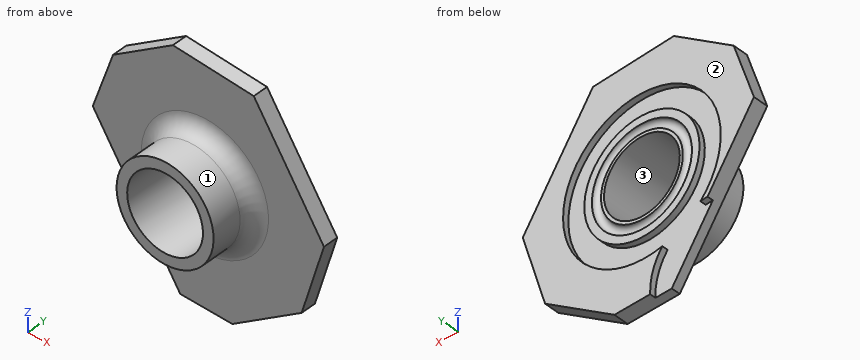
from build123d import *

# Parameters (mm, degrees)
SKETCH_1_R            = 40
SKETCH_1_R_2          = 12.5
EXTRUDE_1_DEPTH       = 20
SKETCH_6_R            = 1.5
SKETCH_12_R           = 43.016285751
SKETCH_12_R_2         = 16
CUT_EXTRUDE_5_DEPTH   = 15
FILLET_2_R            = 5
SKETCH_14_R           = 25.999999999
SKETCH_14_R_2         = 18.999999999
CUT_EXTRUDE_3_DEPTH   = 2
CUT_EXTRUDE_4_DEPTH   = 2
CUT_EXTRUDE_5_2_DEPTH = 10


with BuildPart() as part:
    # Эскиз1 → Вытянуть1 (new body)
    with BuildSketch(Plane(origin=(0, 0, 0), x_dir=(1, 0, 0), z_dir=(0, 1, 0))):
        with Locations(Location((0, 0, 0), (0, 0, 270))):
            Circle(SKETCH_1_R)
        with Locations(Location((0, 0, 0), (0, 0, 270))):
            Circle(SKETCH_1_R_2, mode=Mode.SUBTRACT)
    extrude(amount=EXTRUDE_1_DEPTH)

    # Вырез-По траектории3: sweep along a path in Эскиз4
    with BuildLine(Plane(origin=(0, 20, 0), x_dir=(1, 0, 0), z_dir=(0, 1, 0))) as sweep_3_path:
        CenterArc((0, 0), 15, 0, 360)
    # Эскиз6 → Вырез-По траектории3 (sweep, cut)
    with BuildSketch(Plane(origin=(0, 0, 0), x_dir=(0, 0, -1), z_dir=(1, 0, 0))):
        with Locations((-15, 20)):
            Circle(SKETCH_6_R)
    sweep(path=sweep_3_path.line, mode=Mode.SUBTRACT)

    # Эскиз12 → Cut-Extrude 5 (cut)
    with BuildSketch(Plane.XZ):
        Circle(SKETCH_12_R)
        with Locations(Location((0, 0, 0), (0, 0, 270))):
            Circle(SKETCH_12_R_2, mode=Mode.SUBTRACT)
    extrude(amount=-CUT_EXTRUDE_5_DEPTH, mode=Mode.SUBTRACT)

    # Скругление2
    fillet_2_edges = [part.edges().sort_by_distance(p)[0] for p in [
        (0, 15, 16),
    ]]
    fillet(fillet_2_edges, radius=FILLET_2_R)

    # Эскиз14 → Вырез-Вытянуть3 (cut)
    with BuildSketch(Plane(origin=(0, 20, 0), x_dir=(1, 0, 0), z_dir=(0, 1, 0))):
        with Locations(Location((1.01e-07, 8.4e-08, 0), (0, 0, 270))):
            Circle(SKETCH_14_R)
        with Locations(Location((1.01e-07, 8.4e-08, 0), (0, 0, 270))):
            Circle(SKETCH_14_R_2, mode=Mode.SUBTRACT)
    extrude(amount=-CUT_EXTRUDE_3_DEPTH, mode=Mode.SUBTRACT)

    # Эскиз15 → Вырез-Вытянуть4 (cut)
    with BuildSketch(Plane(origin=(0, 20, 0), x_dir=(1, 0, 0), z_dir=(0, 1, 0))):
        with BuildLine():
            ThreePointArc((-27.297327545, 17.627292527), (-13.760291037, 55.089119116), (-35.71683723, 21.854349851))
            ThreePointArc((-35.71683723, 21.854349851), (-36.252930678, 10.287976674), (-27.297327545, 17.627292527))
        make_face()
    extrude(amount=-CUT_EXTRUDE_4_DEPTH, mode=Mode.SUBTRACT)

    # Эскиз16 → Cut-Extrude 5 2 (cut)
    with BuildSketch(Plane(origin=(0, 20, 0), x_dir=(1, 0, 0), z_dir=(0, 1, 0))):
        Polygon((-7.191454283, -44.519977242), (-37.881198424, -24.469576927), (-45.366952085, 5.371359597), (-23.143023154, 39.387971833), (7.640311576, 44.595915214), (37.770432201, 24.911131357), (45.434410754, -5.233046757), (23.11557492, -39.392615521), align=None)
        Polygon((-8.103935708, 37.866262499), (9.062062667, 38.636931735), (31.933510124, 23.694426018), (39.288073881, -0.614873657), (16.138351941, -36.048532442), (-10.543237541, -38.557583255), (-30.26042154, -25.675839099), (-36.958934768, -6.29707702), align=None, mode=Mode.SUBTRACT)
    extrude(amount=-CUT_EXTRUDE_5_2_DEPTH, mode=Mode.SUBTRACT)


solid = part.part
Input: part model. Units: mm. Frame: model coordinates. Face numbers are marked on the shaded views. Coordinates: 2 decimals unless noted, no trailing zeros. Loops run counter-clockwise (first coordinate to the right, second up) from the corner with the lowest first, then second, coordinate; pieces in that order, holes last.
(1) Pull-direction query (Z, two-part tool) for the marked faces 1, 2 and 3; classes: released by +Z, released by -Z, zero draft, split by the parting line, or undercut.
(2) Section D-D on x = -28.5. Return the cut outline in (y, z).
(3) Material intervals for probe 1 along X at (y, z) = (18.4, 0); probe 2 along X at (y, z) = (9, 0); probe 3 along X at (y, z) = (19.65, 0), sorted ascending.
(4) Section C-C on z = 29.5. Return the cut outline in (x, y).
(5) Section A-A on x = 0. Return the cut outline in (y, z), then the cut area to 3 significant figures.
(6) Section B-B on y = 2. Return the cut outline in (x, z).
(7) First-contact query: pin 1 Ø23 at (x, z) = (0, 8.5) entering from -Y; pin 2 Ø6 at (x, y) = (0, 7) entering from -Z; pin 3 Ø4 at (x, y) = (15.5, 4.5) entering from +Z; pin 4 Ø20 at (x, z) = (0, 0) entering from -Y. Flat tips, straight axial feed; report the tip coordinate or a pass-through.
Data:
1. face 1: split by the parting line
1. face 2: zero draft
1. face 3: undercut
2. outline: (15, -6.65) - (20, -6.65) - (20, 26.83) - (15, 26.83) - close
3. probe 1: x = -32.84 to -26, -19 to -12.5, 12.5 to 19, 26 to 39.1
3. probe 2: x = -16 to -12.5, 12.5 to 16
3. probe 3: x = -32.84 to -26, -19 to -16.46, -13.54 to -12.5, 12.5 to 13.54, 16.46 to 19, 26 to 39.1
4. outline: (-24.41, 15) - (20.42, 15) - (20.42, 20) - (-24.41, 20) - close
5. outline: (0, -16) - (10, -16) arc R5 cw to (15, -21) - (15, -38.23) - (20, -38.23) - (20, -26) - (18, -26) - (18, -19) - (20, -19) - (20, -16.5) arc R1.5 cw to (20, -13.5) - (20, -12.5) - (0, -12.5) - close; (0, 12.5) - (20, 12.5) - (20, 13.5) arc R1.5 cw to (20, 16.5) - (20, 19) - (18, 19) - (18, 26) - (20, 26) - (20, 37.57) - (15, 37.57) - (15, 21) arc R5 cw to (10, 16) - (0, 16) - close
5. area: 335 mm2
6. outline: circle Ø32 at (0, 0); hole circle Ø25 at (0, 0)
7. pin 1: stops at y = 0
7. pin 2: stops at z = -16
7. pin 3: stops at z = 8.59
7. pin 4: passes through
